from build123d import *

# Parameters (mm, degrees)
F0_W     = 8
F0_H     = 16
F1_DEPTH = 10
F2_R     = 2.5
F3_DEPTH = 1
F4_T     = -1.5
F6_DEPTH = 10
F7_R     = 2.3
F7_R_2   = 2.275
F8_DEPTH = 8
F9_DEPTH = 8


with BuildPart() as f1:
    # F0 (on Top) → F1 (new body)
    with BuildSketch(Plane.XY):
        with Locations((-6.5223464929, 11.4436195551)):
            Rectangle(F0_W, F0_H)
    extrude(amount=F1_DEPTH)

    # F2 (on face) → F3 (join)
    with BuildSketch(Plane.XY.offset(10)):
        with Locations((-6.5223464929, 7.4436195551)):
            Circle(F2_R)
        with Locations((-6.5223464929, 15.4436195551)):
            Circle(F2_R)
    extrude(amount=F3_DEPTH)

    # F4
    f4_openings = [f1.faces().sort_by_distance(p)[0] for p in [
        (-6.522346, 11.44362, 0),
    ]]
    offset(amount=F4_T, openings=f4_openings, kind=Kind.INTERSECTION)

    # F5 (on face) → F6 (join)
    with BuildSketch(Plane.XY.offset(10)):
        with BuildLine():
            ThreePointArc((-6.5223464929, 9.9436195551), (-5.4616863211, 10.3829593833), (-5.0223464929, 11.4436195551))
            ThreePointArc((-5.0223464929, 11.4436195551), (-5.4616863203, 12.5042797261), (-6.5223464908, 12.9436195551))
            ThreePointArc((-6.5223464908, 12.9436195551), (-8.0223464929, 11.4436195561), (-6.5223464929, 9.9436195551))
        make_face()
    extrude(amount=-F6_DEPTH)

    # F7 (on face) → F8 (join)
    with BuildSketch(Plane.YZ.offset(-2.5223464929)):
        with Locations((11.4436195551, 5)):
            Circle(F7_R)
        with Locations((11.4436195551, 5)):
            Circle(F7_R_2, mode=Mode.SUBTRACT)
    extrude(amount=-F8_DEPTH)

    # F7 (on face) → F9 (cut)
    with BuildSketch(Plane.YZ.offset(-2.5223464929)):
        with Locations((11.4436195551, 5)):
            Circle(F7_R_2)
    extrude(amount=-F9_DEPTH, mode=Mode.SUBTRACT)


solid = f1.part
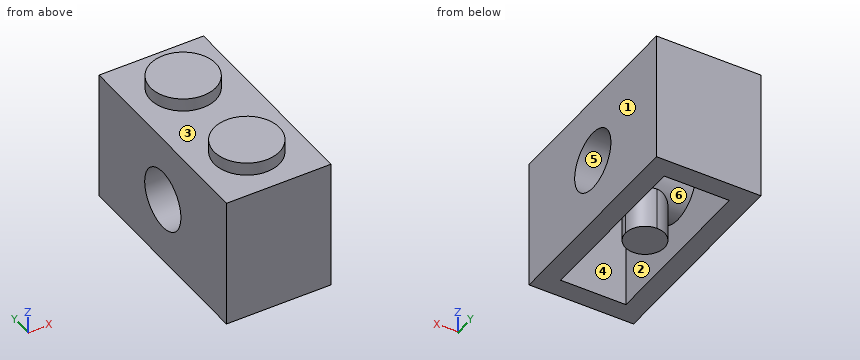
Model file for the job. Use its own axes, mm. Face numbers are marked on the shaded views. A direction names the side the tool comes from. Give positions to 0.01 mm unless a question says otherwise; leave off trailing zeros. Order: outer loops, then holes, each group sorted by start corner. A loop starts at its lowest first (then second) coordinate and runs counter-clockwise, first axis right, second up. Notation, with made-up numbers: M -10.5,-13.75 L 19.5,-13.75 A24 ccw 19.5,-1.75 Z; hole C 0,54.5 d1. An arc over 180 degrees is marked long. Put each result on its own line as item: value. Start each with the question number.
(1) Pull direction X, two halves, no side cores. Call the marked faces 1, 2 and 3: released by +X, released by -X, zero draft, split by the parting line, or undercut.
(2) Band-saw the part on D-D on y = 12.25. Give the cut face in (x, z), then the cut area to 3 significant figures.
(3) Band-saw the part on C-C on x = -8.75. Give the cut face in (y, z) (3 decimals).
(4) Pin check, flat tips, straight feed: pin 1 Ø2 at (x, y) = (-6.5, 15.5) entering from -Z; pin 2 Ø1 at (x, y) = (-4.5, 13) entering from +Z; pin 3 Ø0.6 at (x, y) = (-6.5, 7) entering from -Z. Stop position of each tip, or through.
(5) Band-saw the part on B-B on z = 5. Give the cut face in (x, y), then the cut area to 3 significant figures.
(6) Band-saw the part on A-A on z = 1. Give the cut face in (x, y), then the cut area to 3 significant figures.
(7) Drill centre lines: L1, parallel to Y at x = -6.5, z = 1.5; L2, parallel to X at y = 14.75, z = 5.75; L3, parallel to X at y = 11.75, z = 7.75. Where is each one in solid material? Low to high. Write a range as [from, to].
(8) Tool access for the marked faces 4, 5 and 6: list every direction of +Z, -Z, +X, -X, +Y, -Y with a clear straight run to the whole face (end or side of a thin tool).
Results below:
1. face 1: released by +X
1. face 2: undercut
1. face 3: zero draft
2. outline: M -10.52,0 L -9.02,0 L -9.02,2.85 L -7.79,2.85 L -7.79,0 L -5.26,0 L -5.26,2.85 L -4.02,2.85 L -4.02,0 L -2.52,0 L -2.52,2.87 L -10.52,2.87 Z; M -10.52,7.13 L -2.52,7.13 L -2.52,10 L -10.52,10 Z; hole M -9.02,7.15 L -7.79,7.15 L -7.79,8.5 L -9.02,8.5 Z; hole M -5.26,7.15 L -4.02,7.15 L -4.02,8.5 L -5.26,8.5 Z
2. area: 35.6 mm2
3. outline: M 3.444,0 L 4.944,0 L 4.944,8.5 L 17.944,8.5 L 17.944,0 L 19.444,0 L 19.444,10 L 16.578,10 L 16.578,11 L 14.309,11 L 14.309,10 L 8.578,10 L 8.578,11 L 6.309,11 L 6.309,10 L 3.444,10 Z; C 11.444,5 d4.6; hole C 11.444,5 d4.55
4. pin 1: stops at z = 8.5
4. pin 2: stops at z = 10
4. pin 3: stops at z = 9.5
5. outline: M -10.52,3.44 L -2.52,3.44 L -2.52,9.17 L -10.52,9.17 Z; M -10.52,13.72 L -2.52,13.72 L -2.52,19.44 L -10.52,19.44 Z; hole M -9.02,4.94 L -4.02,4.94 L -4.02,9.14 L -9.02,9.14 Z; hole M -9.02,13.74 L -4.02,13.74 L -4.02,17.94 L -9.02,17.94 Z
5. area: 49.6 mm2
6. outline: M -10.52,3.44 L -2.52,3.44 L -2.52,19.44 L -10.52,19.44 Z; C -6.52,11.44 d3; hole M -9.02,4.94 L -4.02,4.94 L -4.02,17.94 L -9.02,17.94 Z
6. area: 70.1 mm2
7. L1: y = [3.44, 4.94], [9.94, 12.94], [17.94, 19.44]
7. L2: x = [-10.52, -9.02], [-4.02, -2.52]
7. L3: x = [-10.52, -9.02], [-7.99, -5.05], [-4.02, -2.52]
8. face 4: -Z
8. face 5: +X, -X
8. face 6: none
